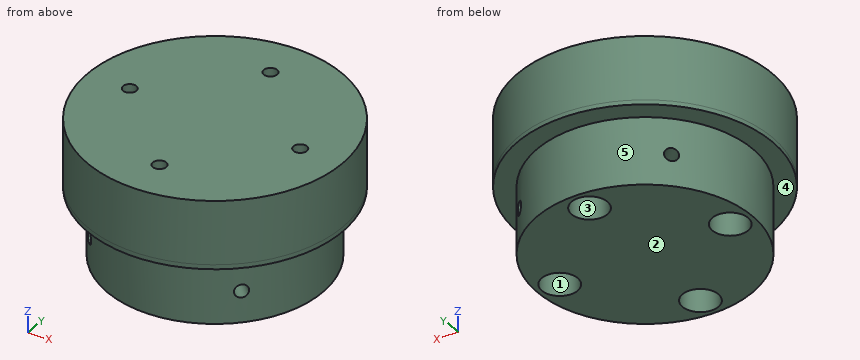
```python
from build123d import *

# Parameters (mm, degrees)
SKETCH_1_R               = 37.5
EXTRUDE_1_DEPTH          = 15.5
SKETCH_2_R               = 3
CUT_EXTRUDE_1_DEPTH      = 16
SKETCH_4_R               = 4.8
CUT_EXTRUDE_2_DEPTH      = 4.5
SKETCH_6_R               = 24.01
EXTRUDE_2_DEPTH          = 23
SKETCH_7_R               = 28.4
EXTRUDE_3_DEPTH          = 14.2
SKETCH_5_R               = 1.5
CUT_EXTRUDE_3_DEPTH      = 33
SKETCH_9_R               = 2.75
CUT_EXTRUDE_6_DEPTH      = 58
EXTRUDE_START            = -1
SKETCH_10_R              = 28.4
EXTRUDE_5_DEPTH          = 1
SKETCH_11_R              = 4
CUT_EXTRUDE_7_DEPTH      = 22
CUT_EXTRUDE_9_DEPTH      = 74
CUT_EXTRUDE_9_DEPTH_BACK = 74
SKETCH_15_R              = 1.45
CUT_EXTRUDE_10_DEPTH     = 74
SKETCH_16_R              = 1.45
CUT_EXTRUDE_11_DEPTH     = 74


with BuildPart() as part:
    # Sketch 1 → Extrude 1 (new body)
    with BuildSketch(Plane.XY):
        Circle(SKETCH_1_R)
    extrude(amount=EXTRUDE_1_DEPTH)

    # Sketch 2 → Cut-Extrude 1 (cut)
    with BuildSketch(Plane(origin=(0, 0, 0), x_dir=(-1, 0, 0), z_dir=(0, 0, -1))):
        with Locations((-25, 0)):
            Circle(SKETCH_2_R)
        with Locations((25, 0)):
            Circle(SKETCH_2_R)
        with Locations((0, 25)):
            Circle(SKETCH_2_R)
        with Locations((0, -25)):
            Circle(SKETCH_2_R)
    extrude(amount=-CUT_EXTRUDE_1_DEPTH, mode=Mode.SUBTRACT)

    # Sketch 4 → Cut-Extrude 2 (cut)
    with BuildSketch(Plane.XY.offset(15.5)):
        with Locations((-25, 0)):
            Circle(SKETCH_4_R)
        with Locations((25, 0)):
            Circle(SKETCH_4_R)
        with Locations((0, 25)):
            Circle(SKETCH_4_R)
        with Locations((0, -25)):
            Circle(SKETCH_4_R)
    extrude(amount=-CUT_EXTRUDE_2_DEPTH, mode=Mode.SUBTRACT)

    # Sketch 6 → Extrude 2 (add)
    with BuildSketch(Plane.XY.offset(15.5)):
        with Locations(Location((0, 0, 0), (0, 0, 168.999166174))):
            Circle(SKETCH_6_R)
    extrude(amount=EXTRUDE_2_DEPTH)

    # Sketch 7 → Extrude 3 (add)
    with BuildSketch(Plane.XY.offset(38.5)):
        Circle(SKETCH_7_R)
    extrude(amount=EXTRUDE_3_DEPTH)

    # Sketch 5 → Cut-Extrude 3 (cut)
    with BuildSketch(Plane.XY.offset(52.7)):
        with Locations((-19, 0)):
            Circle(SKETCH_5_R)
        with Locations((19, 0)):
            Circle(SKETCH_5_R)
        with Locations((0, 19)):
            Circle(SKETCH_5_R)
        with Locations((0, -19)):
            Circle(SKETCH_5_R)
    extrude(amount=-CUT_EXTRUDE_3_DEPTH, mode=Mode.SUBTRACT)

    # Sketch 9 → Cut-Extrude 6 (cut)
    with BuildSketch(Plane(origin=(0, 0, 37.5), x_dir=(-1, 0, 0), z_dir=(0, 0, -1))):
        with Locations(Location((-19, 0, 0), (0, 0, 180))):
            Circle(SKETCH_9_R)
        with Locations(Location((0, 19, 0), (0, 0, 180))):
            Circle(SKETCH_9_R)
        with Locations(Location((19, 0, 0), (0, 0, 180))):
            Circle(SKETCH_9_R)
        with Locations(Location((0, -19, 0), (0, 0, 180))):
            Circle(SKETCH_9_R)
    extrude(amount=CUT_EXTRUDE_6_DEPTH, mode=Mode.SUBTRACT)

    # Sketch 10 → Extrude 5 (add)
    with BuildSketch(Plane(origin=(0, 0, 37.5), x_dir=(-1, 0, 0), z_dir=(0, 0, -1)).offset(EXTRUDE_START)):
        Circle(SKETCH_10_R)
        with BuildLine():
            ThreePointArc((-0.927741091, -20.178684211), (0, -20.5), (0.927741091, -20.178684211))
            ThreePointArc((0.927741091, -20.178684211), (14.28355698, -14.28355698), (20.178684211, -0.927741091))
            ThreePointArc((20.178684211, -0.927741091), (20.5, 0), (20.178684211, 0.927741091))
            ThreePointArc((20.178684211, 0.927741091), (14.28355698, 14.28355698), (0.927741091, 20.178684211))
            ThreePointArc((0.927741091, 20.178684211), (0, 20.5), (-0.927741091, 20.178684211))
            ThreePointArc((-0.927741091, 20.178684211), (-14.28355698, 14.28355698), (-20.178684211, 0.927741091))
            ThreePointArc((-20.178684211, 0.927741091), (-20.5, 0), (-20.178684211, -0.927741091))
            ThreePointArc((-20.178684211, -0.927741091), (-14.28355698, -14.28355698), (-0.927741091, -20.178684211))
        make_face(mode=Mode.SUBTRACT)
    extrude(amount=EXTRUDE_5_DEPTH)

    # Sketch 11 → Cut-Extrude 7 (cut)
    with BuildSketch(Plane(origin=(0, 0, 37.5), x_dir=(-1, 0, 0), z_dir=(0, 0, -1))):
        with Locations(Location((0, 19, 0), (0, 0, 142.890995054))):
            Circle(SKETCH_11_R)
        with Locations(Location((-19, 0, 0), (0, 0, 232.890995054))):
            Circle(SKETCH_11_R)
        with Locations(Location((19, 0, 0), (0, 0, 307.109004946))):
            Circle(SKETCH_11_R)
        with Locations(Location((0, -19, 0), (0, 0, 217.109004946))):
            Circle(SKETCH_11_R)
    extrude(amount=CUT_EXTRUDE_7_DEPTH, mode=Mode.SUBTRACT)

    # Sketch 13 → Cut-Extrude 9 (cut, two sides: drawn at the far end of the back side and taken through both)
    with BuildSketch(Plane(origin=(0, 0, 0), x_dir=(1, 0, 0), z_dir=(0, 1, 0)).offset(-CUT_EXTRUDE_9_DEPTH_BACK)):
        Polygon((-52.212490612, -22.5), (-52.212490612, 12.620192268), (47.798391164, 12.620192268), (47.798391164, -22.5), (0, -22.5), align=None)
    extrude(amount=CUT_EXTRUDE_9_DEPTH + CUT_EXTRUDE_9_DEPTH_BACK, mode=Mode.SUBTRACT)

    # Sketch 15 → Cut-Extrude 10 (cut)
    with BuildSketch(Plane(origin=(16.977633816, -16.977633816, 0), x_dir=(0.7071067811865477, 0.7071067811865475, 0), z_dir=(-0.7071067811865475, 0.7071067811865477, 0))):
        with Locations((0, -29.5)):
            Circle(SKETCH_15_R)
    extrude(amount=CUT_EXTRUDE_10_DEPTH, mode=Mode.SUBTRACT)

    # Sketch 16 → Cut-Extrude 11 (cut)
    with BuildSketch(Plane(origin=(-16.977633816, -16.977633816, 0), x_dir=(0, 0, 1), z_dir=(-0.7071067811865476, -0.7071067811865476, 0))):
        with Locations(Location((29.5, 0, 0), (0, 0, 270))):
            Circle(SKETCH_16_R)
    extrude(amount=-CUT_EXTRUDE_11_DEPTH, mode=Mode.SUBTRACT)


solid = part.part
```
For this review, take the finished solid that the model builds, in its own axes (mm). Face numbers are marked on the shaded views. A direction names the side the tool comes from. Give positions to 0.01 mm unless a question says otherwise; leave off trailing zeros. Order: outer loops, then holes, each group sorted by start corner. A loop starts at its lowest first (then second) coordinate and runs counter-clockwise, first axis right, second up.
1) Take a section at B-B (y = -19). Give the boundary of the cut face in (x, z).
2) Wall thickness on line 1 (X direction, y = 0, z = 44.75); line 2 (X direction, y = -3, z = 25.5): over which ranges is each line inside the solid? List them lowest first.
3) Take a section at A-A (z = 48). Give the boundary of the cut face in (x, y).
4) Take a section at D-D (x = -10). State how many separate pieces and enclosed holes the cut face has, then the cut area to 3 significant figures.
5) For the marked faces 1 and 2, list the 3-axis set-ups (+Z, -Z, +X, -X, +Y, -Y) from which the entire face can be reached by the end or side of a thin tool; tool diameter is ignored.
6) Insertion check: pin 1 (7 mm diameter, centred on x = -19, y = 0, fed in from -Z); pin 2 (4 mm diameter, centred on x = 11, z = 46.5, fed in from +Y); pin 3 (13 mm diameter, centred on x = 0, y = -19, fed in from -Z); pin 4 (1 mm diameter, centred on x = 7.5, z = 46.5, fed in from +Y). Each pin has a flat end and moves straight along its axis. Give the tip position at first contact, or say it passes through.
7) The part is to be moulded in two halves that separate along Y. For the marked faces 3, 4 and 5, say which applies: released by +Y, released by -Y, zero draft, split by the parting line, or undercut.
Derived:
1. outline: (-21.11, 37.5) - (-14.68, 37.5) - (-14.68, 22.5) - (-4, 22.5) - (-4, 37.5) - (-1.5, 37.5) - (-1.5, 52.7) - (-21.11, 52.7) - close; (1.5, 37.5) - (4, 37.5) - (4, 22.5) - (14.68, 22.5) - (14.68, 37.5) - (21.11, 37.5) - (21.11, 52.7) - (1.5, 52.7) - close
2. line 1: x = -28.4 to -20.5, -17.5 to 17.5, 20.5 to 28.4
2. line 2: x = -23.82 to -21.65, -16.35 to 16.35, 21.65 to 23.82
3. outline: circle Ø56.8 at (0, 0); hole circle Ø3 at (-19, 0); hole circle Ø3 at (0, -19); hole circle Ø3 at (0, 19); hole circle Ø3 at (19, 0)
4. separate pieces: 1
4. enclosed holes: 2
4. area: 1,440 mm2
5. face 1: -Z
5. face 2: -Z, +X, -X, +Y, -Y
6. pin 1: stops at z = 37.5
6. pin 2: stops at y = 26.94
6. pin 3: stops at z = 22.5
6. pin 4: stops at y = 27.52
7. face 3: undercut
7. face 4: zero draft
7. face 5: split by the parting line
